Could you check a few things on this drawing? It's one solid part, dimensions in mm from its lowest x, y, z. Coordinates: 2 decimals unless noted, no trailing zeros. Write each loop counter-clockwise with the first axis right and the second up, starting at its lowest first coordinate (ties: lowest second). Pieces come first, ordered by that corner, then holes.
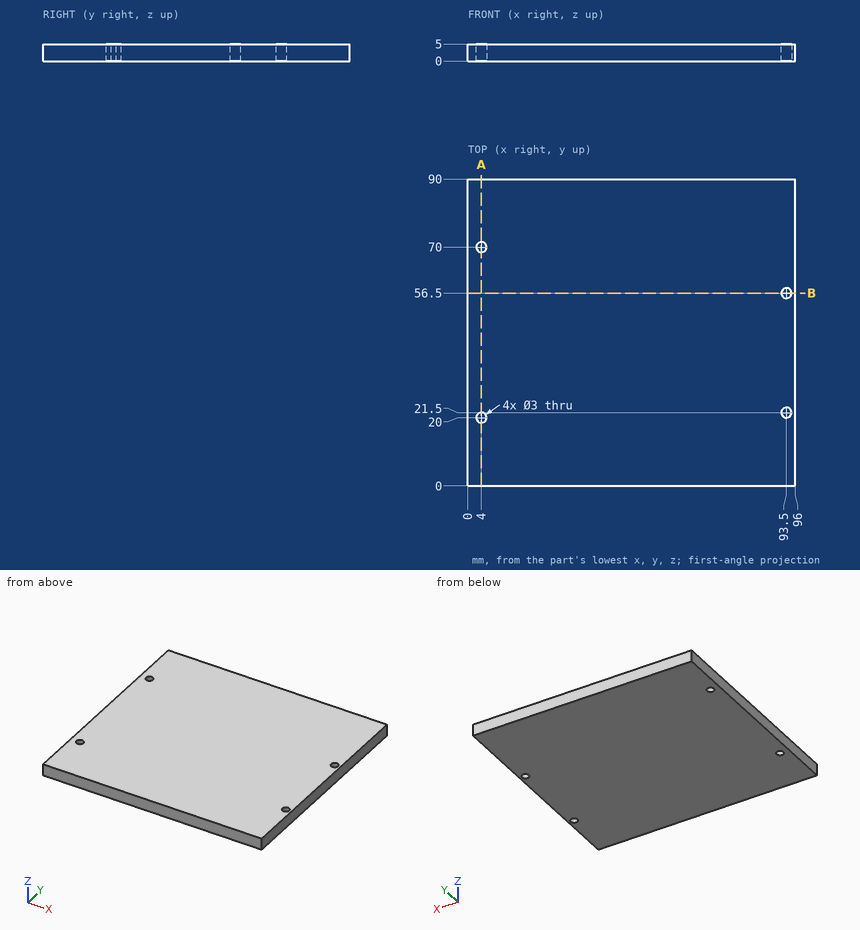
1) Imagine slicing it at B-B on y = 56.5. Please give me the cut outline in (x, z).
Values follow:
outline: (0, 0) - (92, 0) - (92, 5) - (0, 5) - close; (95, 0) - (96, 0) - (96, 5) - (95, 5) - close
2) Will this pin go through, and if not, where does the flat tip stop? pin 1 (2.5 mm diameter, centred on x = 93.5, y = 21.5, fed in from +Z).
Values follow:
pin 1: passes through
3) I need wall thicknesses on probe 1 along Y at (x, z) = (4, 2.1); probe 2 along X at (y, z) = (70, 2.05); probe 3 along Y at (x, z) = (93.5, 3.55). Which ranges of each line are inside material? Lowest first, please.
Values follow:
probe 1: y = 0 to 18.5, 21.5 to 68.5, 71.5 to 90
probe 2: x = 0 to 2.5, 5.5 to 96
probe 3: y = 0 to 20, 23 to 55, 58 to 90
4) Imagine slicing it at A-A on x = 4. Please give me the cut outline in (y, z), then the cut area to 3 significant figures.
Values follow:
outline: (0, 0) - (18.5, 0) - (18.5, 5) - (0, 5) - close; (21.5, 0) - (68.5, 0) - (68.5, 5) - (21.5, 5) - close; (71.5, 0) - (90, 0) - (90, 5) - (71.5, 5) - close
area: 420 mm2
